Check sheet for the modelled part. Datum: model origin and axes. Units: mm. Round coordinates to 2 decimals unless told otherwise and drop trailing zeros. Loops run counter-clockwise (first coordinate to the right, second up) from the corner with the lowest first, then second, coordinate; pieces in that order, holes last. Notation, with made-up numbers: (3, 54) - (55, 54) arc R7 cw to (55, 60) - close; hole circle Ø8 at (62.5, -2). An arc over 180 degrees is marked (long way). Put each result on its own line as item: value. Start each with the question number.
Item 1: Gauge pin test, flat ends, axial feed: pin 1 Ø1 at (y, z) = (69.5, 494.5) entering from -X; pin 2 Ø9.5 at (y, z) = (130.34, 587.46) entering from +X; pin 3 Ø5 at (y, z) = (54, 308.5) entering from -X; pin 4 Ø19 at (y, z) = (130.34, 237.46) entering from +X. Record the tip position at first contact, or that the pin passes through.
Item 2: Section check B-B, the plane y = 165.5. Record the cut outline in (x, z), and give its area (3 significant figures).
Item 3: Section check A-A, the plane y = 53.5. Record the cut outline in (x, z).
Item 4: Material ranges on line 1 along X through (y, z) = (77, 93.5); line 2 along X through (y, z) = (221.5, 518); line 3 along Z through (x, y) = (197.5, 232), recorded low to high.
Item 5: Draft check along Z on faces 1 (the flat face through (126, 0, 414)), 2 (the cylindrical face through (49.559, 134.363, 233.008)), 3 (the flat face through (47, 87, 62.459)). Enter one of: pulls with the +Z half, pulls with the -Z half, needs draft (parallel to the pull), parting line crosses it, or undercut.
from build123d import *

# Parameters (mm, degrees)
REVOLVE1_ANGLE          = 88
CUT_EXTRUDE2_DEPTH      = 2771.780439466
CUT_EXTRUDE2_DEPTH_BACK = 2771.780439466
SKETCH5_W               = 5800.528681758
SKETCH5_H               = 2435.889164845
CUT_EXTRUDE4_DEPTH      = 838.656303446
CUT_EXTRUDE4_DEPTH_BACK = 838.656303446
SKETCH6_R               = 6


with BuildPart() as part:
    # Sketch2 → Revolve1 (revolve)
    with BuildSketch(Plane.XY):
        with BuildLine():
            Line((72.370392529, 0), (82.370392529, 0))
            ThreePointArc((82.370392529, 0), (40.524594063, 121.838677192), (53.578690935, 250))
            Line((53.578690935, 250), (43.578690935, 250))
            ThreePointArc((43.578690935, 250), (31.595154891, 121.961970263), (72.370392529, 0))
        make_face()
    revolve(axis=Axis((2000, -13.371705106, 0), (0, 1, 0)), revolution_arc=REVOLVE1_ANGLE)

    # Sketch5 → Cut-Extrude2 (cut, two sides: drawn at the far end of the back side and taken through both)
    with BuildSketch(Plane(origin=(0, 0, 0), x_dir=(0, 0, -1), z_dir=(1, 0, 0)).offset(-CUT_EXTRUDE2_DEPTH_BACK)):
        with Locations((76.037885341, -87.116535175)):
            Rectangle(SKETCH5_W, SKETCH5_H)
        Polygon((-762.459239957, 250), (-762.459239957, 0), (-62.459239957, 0), (-62.459239957, 175), align=None, mode=Mode.SUBTRACT)
    extrude(amount=CUT_EXTRUDE2_DEPTH + CUT_EXTRUDE2_DEPTH_BACK, mode=Mode.SUBTRACT)

    # Sketch6 → Cut-Extrude4 (cut, two sides: drawn at the far end of the back side and taken through both)
    with BuildSketch(Plane(origin=(0, 0, 0), x_dir=(0, 0, -1), z_dir=(1, 0, 0)).offset(-CUT_EXTRUDE4_DEPTH_BACK)):
        with Locations(Location((-587.459239957, 130.34, 0), (0, 0, 320.485227815))):
            Circle(SKETCH6_R)
        with Locations(Location((-237.459239957, 130.34, 0), (0, 0, 304.628365323))):
            Circle(SKETCH6_R)
    extrude(amount=CUT_EXTRUDE4_DEPTH + CUT_EXTRUDE4_DEPTH_BACK, mode=Mode.SUBTRACT)


solid = part.part
Check result:
1. pin 1: x = 105.55
1. pin 2: through
1. pin 3: x = 70.84
1. pin 4: x = 55.6
2. outline: (30.64, 62.46) - (39.69, 62.46) arc R1961.3 cw to (192.97, 762.46) - (183.15, 762.46) arc R1970.35 ccw to start
2. area: 6,520 mm²
3. outline: (48.46, 62.46) - (57.66, 62.46) arc R1943.34 cw to (212.48, 762.46) - (202.49, 762.46) arc R1952.54 ccw to start
4. line 1: 42.39 to 51.43
4. line 2: 105.73 to 115.64
4. line 3: 748.48 to 762.46
5. face 1: needs draft
5. face 2: undercut
5. face 3: pulls with the -Z half
